Read the model definition and answer for the solid it produces. Units are mm, in the model's axes. Face numbers are marked on the shaded views. A direction names the side the tool comes from. Give positions to 0.01 mm unless a question says otherwise; leave off trailing zeros. Order: outer loops, then holes, each group sorted by start corner. A loop starts at its lowest first (then second) coordinate and runs counter-clockwise, first axis right, second up. Notation, with made-up numbers: (39.25, 33) - (51.25, 33) arc R32 ccw to (51.25, 70) - close; hole circle Ø4 at (31, 51.5). An arc over 180 degrees is marked (long way). Write each question's results on one line, items separated by ' | '. Start each with the question number.
Q1. Flat-ended cylindrical pins translate along their axes: P1, Ø2, axis at y = 2.5, z = 46, coming from the +X side; P2, Ø8, axis at x = 3, y = 9, coming from the -Z side; P3, Ø2, axis at y = 4, z = 39, coming from the -X side; P4, Ø10, axis at x = 2, z = 41, coming from the +Y side. Find the tip coordinate at first contact, or state that the pin passes through.
Q2. Find section A-A on y = 0. Give the vertices of the cut face in (x, z).
Q3. A tool of negligible diameter and unlimited length cuts with its end or side. For the marked faces 1, 2 and 3, from which of +Z, -Z, +X, -X, +Y, -Y can it reach the whole face along a straight path? Write none if from no direction.
Q4. Find section C-C on z = 46.5. Give the vertices of the cut face in (x, y).
Q5. Find the intervals of material crossed by line 1 along Z through (x, y) = (13, 6.5); line 2 along X through (y, z) = (1.5, 46.5); line 3 along Y through (x, z) = (7, 34.5), in increasing order. Write a range as from..to.
Q6. Find section D-D on z = 21.5. Give the vertices of the cut face in (x, y).
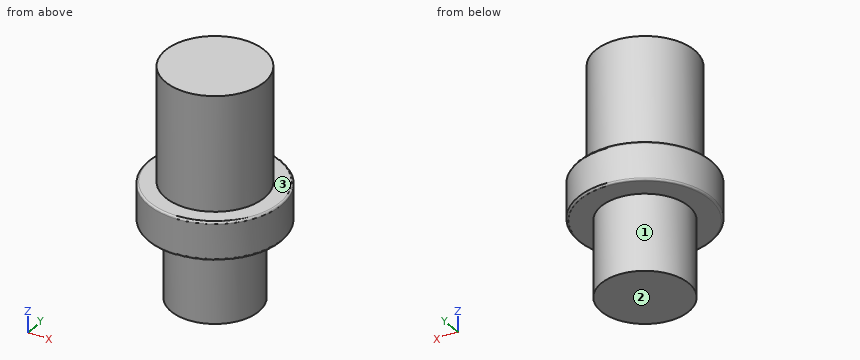
from build123d import *

# Parameters (mm, degrees)
SKETCH1_R           = 11.5
BOSS_EXTRUDE1_DEPTH = 20
SKETCH2_R           = 17.5
BOSS_EXTRUDE2_DEPTH = 10
SKETCH3_R           = 13
BOSS_EXTRUDE3_DEPTH = 30
FILLET1_R           = 0.5


with BuildPart() as part:
    # Sketch1 → Boss-Extrude1 (new body)
    with BuildSketch(Plane.XY):
        Circle(SKETCH1_R)
    extrude(amount=BOSS_EXTRUDE1_DEPTH)

    # Sketch2 → Boss-Extrude2 (add)
    with BuildSketch(Plane.XY.offset(20)):
        Circle(SKETCH2_R)
    extrude(amount=BOSS_EXTRUDE2_DEPTH)

    # Sketch3 → Boss-Extrude3 (add)
    with BuildSketch(Plane.XY.offset(30)):
        Circle(SKETCH3_R)
    extrude(amount=BOSS_EXTRUDE3_DEPTH)

    # Fillet1
    fillet1_edges = [part.edges().sort_by_distance(p)[0] for p in [
        (-17.5, 0, 20),
        (-17.5, 0, 30),
    ]]
    fillet(fillet1_edges, radius=FILLET1_R)


solid = part.part
Working result:
1) P1: x = 12.91 | P2: z = 0 | P3: x = -12.65 | P4: y = 13
2) outline: (-17.5, 20.5) arc R0.5 ccw to (-17, 20) - (-11.5, 20) - (-11.5, 0) - (11.5, 0) - (11.5, 20) - (17, 20) arc R0.5 ccw to (17.5, 20.5) - (17.5, 29.5) arc R0.5 ccw to (17, 30) - (13, 30) - (13, 60) - (-13, 60) - (-13, 30) - (-17, 30) arc R0.5 ccw to (-17.5, 29.5) - close
3) face 1: -Z | face 2: -Z, +X, -X, +Y, -Y | face 3: +Z
4) outline: circle Ø26 at (0, 0)
5) line 1: 20..30 | line 2: -12.91..12.91 | line 3: -10.95..10.95
6) outline: circle Ø35 at (0, 0)
